Part model, mm, in its own coordinate system. Face numbers are marked on the shaded views. A direction names the side the tool comes from. Round coordinates to 2 decimals unless told otherwise and drop trailing zeros. Order: outer loops, then holes, each group sorted by start corner. A loop starts at its lowest first (then second) coordinate and runs counter-clockwise, first axis right, second up. Notation, with made-up numbers: (62.5, 21) -> (92.5, 21) arc R10 ccw to (92.5, 31) -> close; hole circle Ø6 at (60, 89). An arc over 180 degrees is marked (long way). Answer as a JSON object with one key per item and string values. Group by question number.
```python
from build123d import *

# Parameters (mm, degrees)
SKETCH1_R               = 4.625
BOSS_EXTRUDE1_DEPTH     = 10
BOSS_EXTRUDE2_DEPTH     = 42.94
BOSS_EXTRUDE3_DEPTH     = 17.14
CUT_EXTRUDE1_DEPTH      = 123.845099649
CUT_EXTRUDE1_DEPTH_BACK = 123.845099649
SKETCH4_R               = 0.75


with BuildPart() as part:
    # Sketch1 → Boss-Extrude1 (new body)
    with BuildSketch(Plane.XY):
        with BuildLine():
            Line((-7.5, 50.8), (-7.5, -50.8))
            ThreePointArc((-7.5, -50.8), (0, -58.3), (7.5, -50.8))
            Line((7.5, -50.8), (7.5, 50.8))
            ThreePointArc((7.5, 50.8), (0, 43.3), (-7.5, 50.8))
        make_face()
        with Locations((0, -50.8)):
            Circle(SKETCH1_R, mode=Mode.SUBTRACT)
        with BuildLine():
            ThreePointArc((5, -34.675), (0, -39.675), (-5, -34.675))
            Line((-5, -34.675), (-5, -9.675))
            ThreePointArc((-5, -9.675), (0, -4.675), (5, -9.675))
            Line((5, -9.675), (5, -34.675))
        make_face(mode=Mode.SUBTRACT)
        with BuildLine():
            ThreePointArc((-5, 31.8), (0, 36.8), (5, 31.8))
            Line((5, 31.8), (5, 6.8))
            ThreePointArc((5, 6.8), (0, 1.8), (-5, 6.8))
            Line((-5, 6.8), (-5, 31.8))
        make_face(mode=Mode.SUBTRACT)
    extrude(amount=BOSS_EXTRUDE1_DEPTH)

    # Sketch1_4 → Boss-Extrude2 (add)
    with BuildSketch(Plane.XY):
        with BuildLine():
            ThreePointArc((7.5, 50.8), (0, 58.3), (-7.5, 50.8))
            ThreePointArc((-7.5, 50.8), (0, 43.3), (7.5, 50.8))
        make_face()
    extrude(amount=BOSS_EXTRUDE2_DEPTH)

    # Sketch3 → Boss-Extrude3 (add)
    with BuildSketch(Plane.XY.offset(42.94)):
        Polygon((0, 43.3), (6.495190528, 47.05), (6.495190528, 54.55), (0, 58.3), (-6.495190528, 54.55), (-6.495190528, 47.05), align=None)
    extrude(amount=BOSS_EXTRUDE3_DEPTH)

    # Sketch4 → Cut-Extrude1 (cut, two sides: drawn at the far end of the back side and taken through both)
    with BuildSketch(Plane(origin=(25.24464052, 43.725, 0), x_dir=(0.8660254037844416, -0.499999999999995, 0), z_dir=(0.49999999999999495, 0.8660254037844415, 0)).offset(-CUT_EXTRUDE1_DEPTH_BACK)):
        with Locations(Location((-25.4, -56.83, 0), (0, 0, 180))):
            Circle(SKETCH4_R)
    extrude(amount=CUT_EXTRUDE1_DEPTH + CUT_EXTRUDE1_DEPTH_BACK, mode=Mode.SUBTRACT)


solid = part.part
```
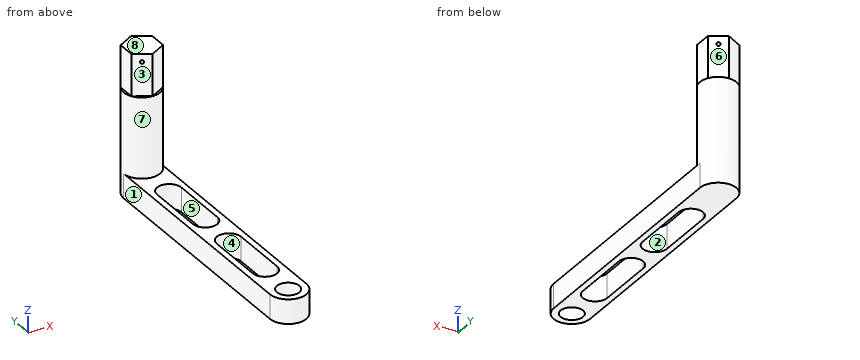
Q1. Band-saw the part on B-B (z = 54). List the corners of the cut face in (x, y), plus the area to 3 significant figures.
Q2. Which spindle directions (+Z, -Z, +X, -X, +Y, -Y) get a long thin tool onto all of the face, cutting with end or side? Do the marked faces 5, 6, 7 and 8. Say none if no direction does.
Q3. Band-saw the part on C-C (z = 40.5). List the corners of the cut face in (x, y), plus the area to 3 significant figures.
Q4. Band-saw the part on A-A (y = 18). List the corners of the cut face in (x, z), plus the area to 3 significant figures.
Q5. Wall check: line 1 (Y direction, x = 0, z = 4.75) (3 decimals); line 2 (X direction, y = -32.5, z = 4.5); line 3 (Z direction, x = 6.75, y = -14.5). Give the ranges that are in metal, low to high. Write a range as [from, to].
Q6. Two-plate mould, pull along Y, no slides. Class the marked faces 1, 2, 3 and 4: +Y half, -Y half, draft (parallel to the pull), parting line (faces both ways), or undercut.
Q7. Drop flat-ended pins along their axis: pin 1 Ø8 at (x, z) = (4.5, 12) entering from -Y; pin 2 Ø1.1 at (x, y) = (3.5, 44.5) entering from +Z; pin 3 Ø8 at (x, z) = (-5, 42) entering from -Y. Give the stop position or say it passes through.
Completed:
{
 "1": {"outline": "(-6.5, 47.05) -> (0, 43.3) -> (6.5, 47.05) -> (6.5, 54.55) -> (0, 58.3) -> (-6.5, 54.55) -> close", "area": "146 mm2"},
 "2": {"face 5": "+Z, -Z", "face 6": "+Z, +X, +Y", "face 7": "+Z", "face 8": "+Z, +X, -X, +Y, -Y"},
 "3": {"outline": "circle Ø15 at (0, 50.8)", "area": "177 mm2"},
 "4": {"outline": "(-7.5, 0) -> (-5, 0) -> (-5, 10) -> (-7.5, 10) -> close; (5, 0) -> (7.5, 0) -> (7.5, 10) -> (5, 10) -> close", "area": "50.0 mm2"},
 "5": {"line 1": "[-58.3, -55.425], [-46.175, -39.675], [-4.675, 1.8], [36.8, 58.3]", "line 2": "[-7.5, -5], [5, 7.5]", "line 3": "[0, 10]"},
 "6": {"face 1": "draft", "face 2": "undercut", "face 3": "-Y half", "face 4": "undercut"},
 "7": {"pin 1": "y = -58.23", "pin 2": "z = 42.94", "pin 3": "y = 43.37"}
}
